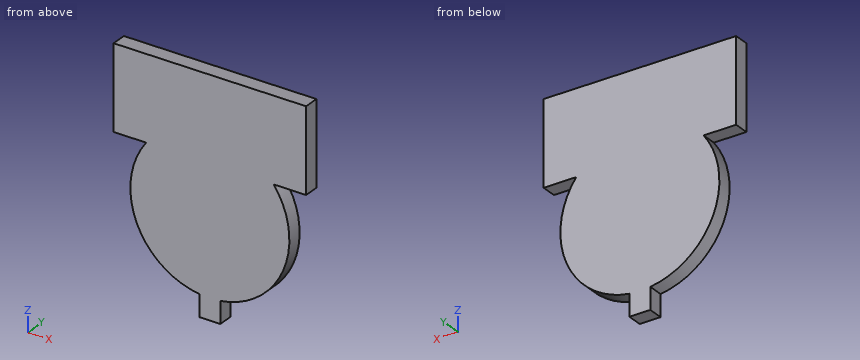
from build123d import *

# Parameters (mm, degrees)
BOSS_EXTRUDE1_DEPTH = 4.572


with BuildPart() as part:
    # Sketch1 → Boss-Extrude1 (new body)
    with BuildSketch(Plane(origin=(0, 0, 0), x_dir=(1, 0, 0), z_dir=(0, 1, 0))):
        with BuildLine():
            Line((-3.175, 30.524206416), (3.175, 30.524206416))
            Line((3.175, 30.524206416), (3.175, 23.920206416))
            ThreePointArc((3.175, 23.920206416), (22.234995228, 9.373467192), (19.341279759, -14.428159872))
            Line((19.341279759, -14.428159872), (29.21, -14.428159872))
            Line((29.21, -14.428159872), (29.21, -39.828159872))
            Line((29.21, -39.828159872), (-29.21, -39.828159872))
            Line((-29.21, -39.828159872), (-29.21, -14.428159872))
            Line((-29.21, -14.428159872), (-19.341279759, -14.428159872))
            ThreePointArc((-19.341279759, -14.428159872), (-22.234995228, 9.373467192), (-3.175, 23.920206416))
            Line((-3.175, 23.920206416), (-3.175, 30.524206416))
        make_face()
    extrude(amount=BOSS_EXTRUDE1_DEPTH)


solid = part.part
Verification items for the finished model (mm, model axes). Coordinates: 2 decimals unless noted, no trailing zeros. Order: outer loops, then holes, each group sorted by start corner. A loop starts at its lowest first (then second) coordinate and runs counter-clockwise, first axis right, second up.
Item 1: Section check A-A, the plane x = 21.5. Enter the section's corners in (y, z).
Filled in:
outline: (0, -10.95) - (4.57, -10.95) - (4.57, 10.95) - (0, 10.95) - close; (0, 14.43) - (4.57, 14.43) - (4.57, 39.83) - (0, 39.83) - close
Item 2: Section check C-C, the plane z = -25. Enter the section's corners in (x, y) (3 decimals), then the cut area to 3 significant figures.
Filled in:
outline: (-3.175, 0) - (3.175, 0) - (3.175, 4.572) - (-3.175, 4.572) - close
area: 29.0 mm2
Item 3: Section check D-D, the plane x = -6.5. Enter the section's corners in (y, z).
Filled in:
outline: (0, -23.24) - (4.57, -23.24) - (4.57, 39.83) - (0, 39.83) - close
Item 4: Material ranges on L1, parallel to Z at x = -24.5, y = 4.2; L2, parallel to Z at x = 22, y = 4.1; L3, parallel to X at y = 2.8, z = -0.5, recorded low to high.
Filled in:
L1: z = 14.43 to 39.83
L2: z = -9.91 to 9.91, 14.43 to 39.83
L3: x = -24.12 to 24.12
Item 5: Section check B-B, the plane y = 1.7. Enter the section's corners in (x, z) (3 decimals), then the cut area to 3 significant figures.
Filled in:
outline: (-29.21, 14.428) - (-19.341, 14.428) arc R24.13 ccw to (-3.175, -23.92) - (-3.175, -30.524) - (3.175, -30.524) - (3.175, -23.92) arc R24.13 ccw to (19.341, 14.428) - (29.21, 14.428) - (29.21, 39.828) - (-29.21, 39.828) - close
area: 3,090 mm2
Item 6: Depth check by flat-ended pin: pin 1 (1 mm diameter, centred on y = 0.5, z = 8.5, fed in from -X); pin 2 (1.4 mm diameter, centred on y = 3, z = -25.5, fed in from -X) (3 decimals). Enter the tip coordinate at first touch or a pass-through.
Filled in:
pin 1: stops at x = -22.77
pin 2: stops at x = -3.175
